Could you check a few things on this model? Use its own coordinates, in mm. A direction names the side the tool comes from. Give positions to 0.01 mm unless a question says otherwise; leave off trailing zeros. Write each loop counter-clockwise with the first axis right and the second up, starting at its lowest first coordinate (ties: lowest second). Pieces come first, ordered by that corner, then holes. Notation, with made-up numbers: (12, 32.25) - (53, 32.25) arc R7 cw to (53, 40.25) - close; hole circle Ø9 at (-27, 4). An arc over 180 degrees is marked (long way). Write item = value, one per line.
from build123d import *

# Parameters (mm, degrees)
SKETCH1_W           = 65
SKETCH1_H           = 55
BOSS_EXTRUDE1_DEPTH = 44
SKETCH2_W           = 39
SKETCH2_H           = 20
CUT_EXTRUDE1_DEPTH  = 96.843622636
FILLET1_R           = 5
SKETCH3_R           = 3.1
CUT_EXTRUDE2_DEPTH  = 8.5
SKETCH4_R           = 3.1
CUT_EXTRUDE3_DEPTH  = 10
FILLET2_R           = 5


with BuildPart() as part:
    # Sketch1 → Boss-Extrude1 (new body)
    with BuildSketch(Plane(origin=(0, 0, 0), x_dir=(1, 0, 0), z_dir=(0, 1, 0))):
        with Locations((32.5, 27.5)):
            Rectangle(SKETCH1_W, SKETCH1_H)
    extrude(amount=BOSS_EXTRUDE1_DEPTH)

    # Sketch2 → Cut-Extrude1 (cut, through all)
    with BuildSketch(Plane.XY):
        with Locations((32.5, 10)):
            Rectangle(SKETCH2_W, SKETCH2_H)
    extrude(amount=-CUT_EXTRUDE1_DEPTH, mode=Mode.SUBTRACT)

    # Fillet1
    fillet1_edges = [part.edges().sort_by_distance(p)[0] for p in [
        (52, 20, -27.5),
        (13, 20, -27.5),
    ]]
    fillet(fillet1_edges, radius=FILLET1_R)

    # Sketch3 → Cut-Extrude2 (cut)
    with BuildSketch(Plane.XZ):
        with Locations(Location((58.5, -6.5, 0), (0, 0, 270))):
            Circle(SKETCH3_R)
        with Locations(Location((58.5, -48.5, 0), (0, 0, 270))):
            Circle(SKETCH3_R)
        with Locations(Location((6.5, -48.5, 0), (0, 0, 270))):
            Circle(SKETCH3_R)
        with Locations(Location((6.5, -6.5, 0), (0, 0, 270))):
            Circle(SKETCH3_R)
    extrude(amount=-CUT_EXTRUDE2_DEPTH, mode=Mode.SUBTRACT)

    # Sketch4 → Cut-Extrude3 (cut)
    with BuildSketch(Plane(origin=(0, 44, 0), x_dir=(1, 0, 0), z_dir=(0, 1, 0))):
        with Locations(Location((10, 45, 0), (0, 0, 270))):
            Circle(SKETCH4_R)
        with Locations(Location((55, 45, 0), (0, 0, 270))):
            Circle(SKETCH4_R)
        with Locations(Location((55, 10, 0), (0, 0, 270))):
            Circle(SKETCH4_R)
        with Locations(Location((10, 10, 0), (0, 0, 270))):
            Circle(SKETCH4_R)
    extrude(amount=-CUT_EXTRUDE3_DEPTH, mode=Mode.SUBTRACT)

    # Fillet2
    fillet2_edges = [part.edges().sort_by_distance(p)[0] for p in [
        (0, 22, -55),
        (65, 22, -55),
        (65, 22, 0),
        (0, 22, 0),
    ]]
    fillet(fillet2_edges, radius=FILLET2_R)


solid = part.part
1. Thinking about a two-plate mould opening in Z: for faces 1 (the face through (10, 34, -45)), 2 (the face through (1, 22, -53)), 3 (the face through (52, 7, -27)), which applies, pulls with the +Z half, pulls with the -Z half, needs draft (parallel to the pull), parting line crosses it, or undercut?
Filled sheet:
face_1 = undercut
face_2 = pulls with the -Z half
face_3 = needs draft
2. If we section it at C-C, the plane y = 41: Please give me the cut outline in (x, z).
Filled sheet:
outline = (0, -50) arc R5 ccw to (5, -55) - (60, -55) arc R5 ccw to (65, -50) - (65, -5) arc R5 ccw to (60, 0) - (5, 0) arc R5 ccw to (0, -5) - close; hole circle Ø6.2 at (10, -45); hole circle Ø6.2 at (10, -10); hole circle Ø6.2 at (55, -45); hole circle Ø6.2 at (55, -10)
3. For pin 1 (2 mm diameter, centred on x = 39, z = -48, fed in from -Y); pin 2 (3.5 mm diameter, centred on x = 10, z = -10, fed in from +Y), each with a flat end and sliding along its axis, tell me the tip position at first contact or that it passes through.
Filled sheet:
pin_1 = 20
pin_2 = 34
4. If we section it at B-B, the plane z = -20.5: Please give me the cut outline in (x, y), and give its area (3 significant figures).
Filled sheet:
outline = (0, 0) - (13, 0) - (13, 15) arc R5 cw to (18, 20) - (47, 20) arc R5 cw to (52, 15) - (52, 0) - (65, 0) - (65, 44) - (0, 44) - close
area = 2,090 mm2
5. If we section it at A-A, the plane y = 5: Please give me the cut outline in (x, z), and give its area (3 significant figures).
Filled sheet:
outline = (0, -50) arc R5 ccw to (5, -55) - (13, -55) - (13, 0) - (5, 0) arc R5 ccw to (0, -5) - close; (52, -55) - (60, -55) arc R5 ccw to (65, -50) - (65, -5) arc R5 ccw to (60, 0) - (52, 0) - close; hole circle Ø6.2 at (6.5, -48.5); hole circle Ø6.2 at (6.5, -6.5); hole circle Ø6.2 at (58.5, -48.5); hole circle Ø6.2 at (58.5, -6.5)
area = 1,290 mm2
6. Which directions (+Z, -Z, +X, -X, +Y, -Y) give clear straight access to the entire face, cutting with the end or side of a thin tool? Please do faces 4 (the face through (13, 7, -27)), 5 (the face through (61.574, 4.19, -48.096)), 6 (the face through (55, 34, -45)).
Filled sheet:
face_4 = +Z, -Z, -Y
face_5 = -Y
face_6 = +Y
7. I need wall thicknesses on line 1 (X direction, y = 6.75, z = -48.5); line 2 (X direction, y = 40, z = -45); line 3 (Z direction, x = 6, y = 6). Which ranges of each line are inside material? Lowest first, please.
Filled sheet:
line_1 = 0 to 3.4, 9.6 to 13, 52 to 55.4, 61.6 to 65
line_2 = 0 to 6.9, 13.1 to 51.9, 58.1 to 65
line_3 = -55 to -51.56, -45.44 to -9.56, -3.44 to 0
8. If we section it at D-D, the plane x = 39.5: Please give me the cut outline in (y, z), and give its area (3 significant figures).
Filled sheet:
outline = (20, -55) - (44, -55) - (44, 0) - (20, 0) - close
area = 1,320 mm2
